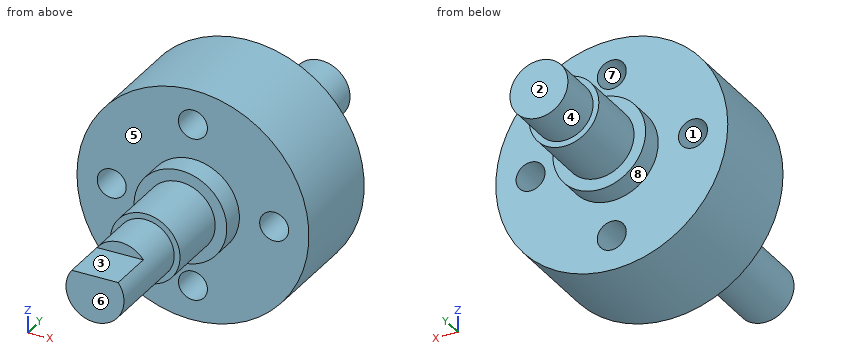
from build123d import *

# Parameters (mm, degrees)
HOLE_WIZARD_M3_1_D       = 2.5
PATTERN_CIRCULAR_1_COUNT = 4
CUT_EXTRUDE_1_DEPTH      = 4


with BuildPart() as part:
    # Model → 旋转1 (revolve)
    with BuildSketch(Plane.XY, mode=Mode.PRIVATE) as revolve_1_sk:
        Polygon((-1.786351506, 30.377960803), (-1.786351506, -5.622039197), (0.713648494, -5.622039197), (0.713648494, 2.377960803), (1.213648494, 2.377960803), (1.213648494, 7.977960803), (2.213648494, 7.977960803), (2.213648494, 9.977960803), (8.213648494, 9.977960803), (8.213648494, 18.777960803), (2.213648494, 18.777960803), (2.213648494, 20.777960803), (1.213648494, 20.777960803), (1.213648494, 26.377960803), (0.713648494, 26.377960803), (0.713648494, 30.377960803), align=None)
    revolve(revolve_1_sk.sketch.rotate(Axis((-1.786351506, 30.377960803, 0), (0, -1, 0)), 180), axis=Axis((-1.786351506, 30.377960803, 0), (0, -1, 0)))

    # M3 螺纹孔1 (through all)
    with Locations(Plane(origin=(-1.786351506, 9.977960803, 7), x_dir=(-1, 0, 0), z_dir=(0, -1, 0))):
        with Locations((0, 0)):
            hole_wizard_m3_1 = Hole(HOLE_WIZARD_M3_1_D / 2)

    # 阵列(圆周)1: M3 螺纹孔1 ×4 about axis
    pattern_circular_1_axis = Axis((-1.786351506, 0, 0), (0, 1, 0))
    for i in range(1, PATTERN_CIRCULAR_1_COUNT):
        add(hole_wizard_m3_1.rotate(pattern_circular_1_axis, i * 360 / PATTERN_CIRCULAR_1_COUNT), mode=Mode.SUBTRACT)

    # 草图5 → 切除-拉伸1 (cut)
    with BuildSketch(Plane.XZ.offset(5.622039197)):
        Polygon((-3.786351506, 1.5), (0.213648494, 1.5), (0.213648494, 5.333306347), (-4.133002322, 4.430820446), align=None)
    extrude(amount=-CUT_EXTRUDE_1_DEPTH, mode=Mode.SUBTRACT)


solid = part.part
Could you check a few things on this model? Use its own coordinates, in mm. Face numbers are marked on the shaded views. A direction names the side the tool comes from. Give positions to 0.01 mm unless a question says otherwise; leave off trailing zeros. Order: outer loops, then holes, each group sorted by start corner. A loop starts at its lowest first (then second) coordinate and runs counter-clockwise, first axis right, second up. Notation, with made-up numbers: (64, -19.5) - (75, -19.5) arc R13 cw to (75, -4.5) - close; hole circle Ø1 at (33.25, -14.5). An arc over 180 degrees is marked (long way). One line per question, with ' | ' between items. Start each with the question number.
Item 1: Thinking about a two-plate mould opening in Z: for the marked faces 6, 7 and 8, which applies, pulls with the +Z half, pulls with the -Z half, needs draft (parallel to the pull), parting line crosses it, or undercut?
Item 2: I need wall thicknesses on probe 1 along Y at (x, z) = (1.5, 9); probe 2 along Y at (x, z) = (0.5, 1.5); probe 3 along X at (y, z) = (16.25, 7). Which ranges of each line are inside material? Lowest first, please. Write a range as [from, to].
Item 3: I want a section at B-B on x = -9.25. Write out the boundary of the cut face in (y, z).
Item 4: I want a section at C-C on z = 0. Give the number of separate pieces and of enclosed holes in the cut face, then the cut area to 3 significant figures.
Item 5: I want a section at A-A on z = 7. Write out the boundary of the cut face in (x, y).
Item 6: I'm going to push flat-ended pins straight in: pin 1 Ø12 at (y, z) = (2.5, -1.5) entering from -X; pin 2 Ø6 at (x, y) = (6, 11) entering from +Z; pin 3 Ø2 at (x, z) = (-5, 2) entering from +Y; pin 4 Ø1.5 at (x, z) = (-1.79, 7) entering from -Y. Where does each tip first touch, or does it pass through?
Item 7: I want a section at D-D on y = 11.5. Write out the boundary of the cut face in (x, z), then the cut area to 3 significant figures.
Item 8: For the marked faces 1, 2, 3, 4 and 5, which set-ups out of +Z, -Z, +X, -X, +Y, -Y let a thin tool reach every point of the face, with its end or its side?
Verdict:
1) face 6: needs draft | face 7: undercut | face 8: parting line crosses it
2) probe 1: [9.98, 18.78] | probe 2: [2.38, 26.38] | probe 3: [-8.93, -3.04], [-0.54, 5.36]
3) outline: (9.98, -6.66) - (18.78, -6.66) - (18.78, -1.16) - (9.98, -1.16) - close; (9.98, 1.16) - (18.78, 1.16) - (18.78, 6.66) - (9.98, 6.66) - close
4) separate pieces: 3 | enclosed holes: 0 | area: 291 mm^2
5) outline: (-8.93, 9.98) - (-3.04, 9.98) - (-3.04, 18.78) - (-8.93, 18.78) - close; (-0.54, 9.98) - (5.36, 9.98) - (5.36, 18.78) - (-0.54, 18.78) - close
6) pin 1: x = -5.79 | pin 2: z = 8.78 | pin 3: y = 26.38 | pin 4: through
7) outline: circle Ø20 at (-1.79, 0); hole circle Ø2.5 at (-8.79, 0); hole circle Ø2.5 at (-1.79, -7); hole circle Ø2.5 at (-1.79, 7); hole circle Ø2.5 at (5.21, 0) | area: 295 mm^2
8) face 1: +Y, -Y | face 2: +Z, -Z, +X, -X, +Y | face 3: +Z, +X, -X, -Y | face 4: +Y | face 5: -Y
